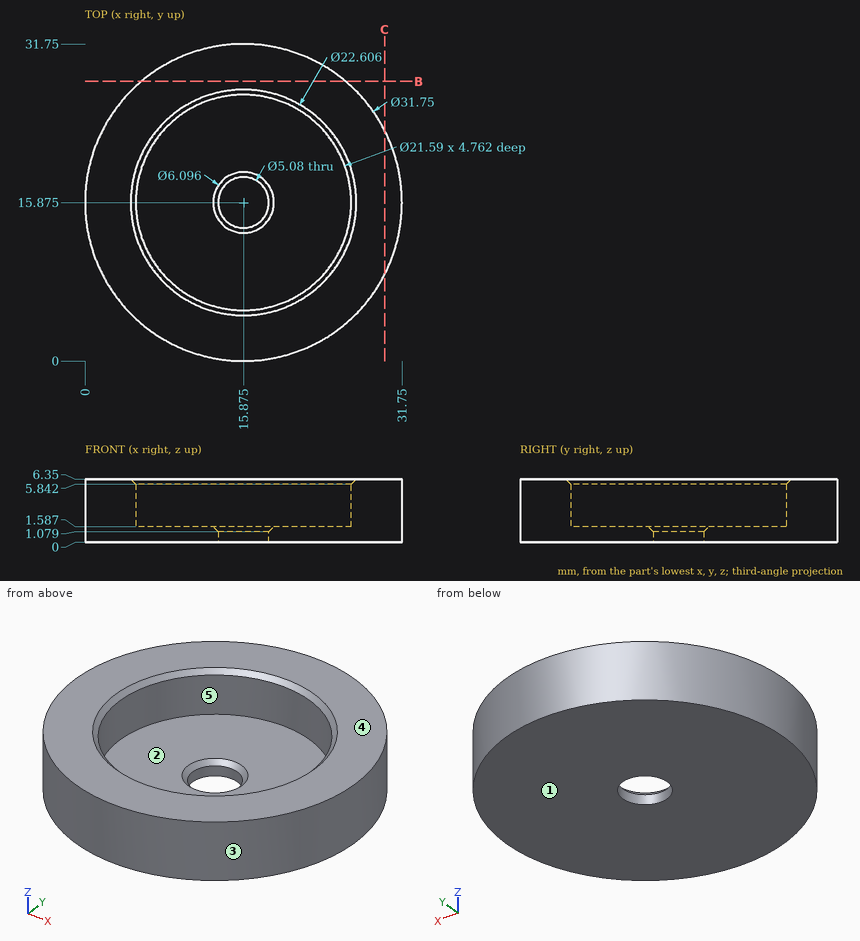
Job drawing, mm, ordinate dimensions from the low corner. One solid piece. A direction names the side the tool comes from. Coordinates: 2 decimals unless noted, no trailing zeros. Write each loop counter-clockwise with the first axis right and the second up, starting at its lowest first coordinate (ties: lowest second). Pieces come first, ordered by that corner, then holes.
Item 1: Pin check, flat tips, straight feed: pin 1 (3 mm diameter, centred on x = 15.875, y = 15.875, fed in from -Z); pin 2 (6.5 mm diameter, centred on x = 15.5, y = 14, fed in from +Z); pin 3 (2 mm diameter, centred on x = 18.5, z = 1, fed in from +Y); pin 4 (3 mm diameter, centred on x = 27, z = 3, fed in from +Y). Stop position of each tip, or through.
Item 2: Which spindle directions (+Z, -Z, +X, -X, +Y, -Y) get a long thin tool onto all of the face, cutting with end or side? Do the marked faces 4 and 5. Say none if no direction does.
Item 3: Probe line 1 (X direction, y = 10, z = 6) (1 decimal); line 2 (X direction, y = 20.5, z = 4.25); line 3 (Z direction, x = 25, y = 15.5). List the from-to ranges inside material, lowest first.
Item 4: Slice it at C-C (x = 30). Write the cut outline in (y, z).
Item 5: Slice it at B-B (y = 28). Write the cut outline in (x, z).
Item 6: Mould opens along Y. For the marked faces 1, 2 and 3 say: released by +Y, released by -Y, zero draft, split by the parting line, or undercut.
Results found:
1. pin 1: passes through
1. pin 2: stops at z = 1.59
1. pin 3: stops at y = 31.67
1. pin 4: stops at y = 28.5
2. face 4: +Z, +X, -X, +Y, -Y
2. face 5: +Z
3. line 1: x = 1.1 to 6.6, 25.1 to 30.6
3. line 2: x = 0.69 to 6.12, 25.63 to 31.06
3. line 3: z = 0 to 1.59
4. outline: (8.63, 0) - (23.12, 0) - (23.12, 6.35) - (8.63, 6.35) - close
5. outline: (5.63, 0) - (26.12, 0) - (26.12, 6.35) - (5.63, 6.35) - close
6. face 1: zero draft
6. face 2: undercut
6. face 3: split by the parting line
